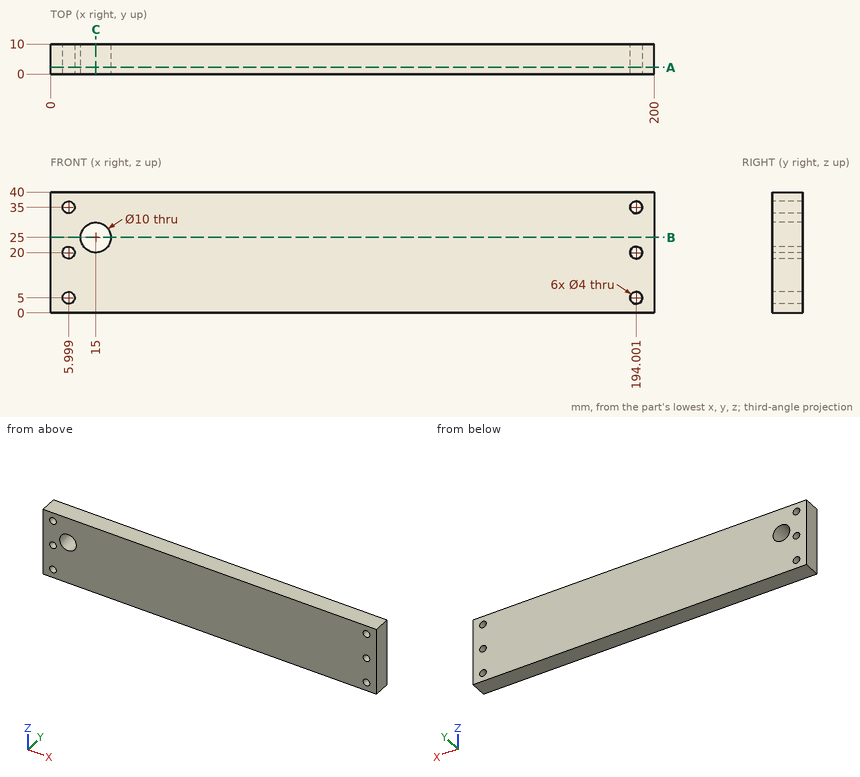
Study the drawing (mm; zero at the part's minimum x, y, z) and answer. Give positions to 0.01 mm unless a question says otherwise; leave off trailing zeros. Write each loop counter-clockwise with the first axis right and the second up, starting at its lowest first coordinate (ties: lowest second). Pieces come first, ordered by that corner, then holes. Notation, with made-up numbers: (-28.75, 36) -> (-6.75, 36) arc R18 ccw to (-6.75, 54) -> close; hole circle Ø6 at (55.25, 29). An arc over 180 degrees is marked (long way). Answer in a Markdown table with one row per item.
1) Section C-C on x = 15 is taken. Give the vertices of the cut face in (y, z).
Results list:
| item | result |
|---|---|
| outline | (0, 0) -> (10, 0) -> (10, 20) -> (0, 20) -> close; (0, 30) -> (10, 30) -> (10, 40) -> (0, 40) -> close |
2) Section B-B on z = 25 is taken. Give the vertices of the cut face in (x, y), plus the area to 3 significant figures.
Results list:
| item | result |
|---|---|
| outline | (0, 0) -> (10, 0) -> (10, 10) -> (0, 10) -> close; (20, 0) -> (200, 0) -> (200, 10) -> (20, 10) -> close |
| area | 1,900 mm^2 |
3) Straight lines are drawn through the part: line 1 (X direction, y = 5.5, z = 3.5) (1 decimal); line 2 (X direction, y = 4.75, z = 35.5) (1 decimal); line 3 (X direction, y = 1.25, z = 29.5). For each, find the intervals that lie inside material, in ascending order. Write a range as [from, to].
Results list:
| item | result |
|---|---|
| line 1 | [0, 4.7], [7.3, 192.7], [195.3, 200] |
| line 2 | [0, 4.1], [7.9, 192.1], [195.9, 200] |
| line 3 | [0, 12.82], [17.18, 200] |
4) Section A-A on y = 2.25 is taken. Give the vertices of the cut face in (x, z).
Results list:
| item | result |
|---|---|
| outline | (0, 0) -> (200, 0) -> (200, 40) -> (0, 40) -> close; hole circle Ø4 at (6, 5); hole circle Ø4 at (6, 20); hole circle Ø4 at (6, 35); hole circle Ø10 at (15, 25); hole circle Ø4 at (194, 5); hole circle Ø4 at (194, 20); hole circle Ø4 at (194, 35) |
5) Each of these flat-tipped pins is pushed along its axis until it touches: pin 1 Ø6 at (y, z) = (5.5, 19) entering from -X; pin 2 Ø3.5 at (x, z) = (6, 35) entering from -Y. Where does it stop, or does it pass through?
Results list:
| item | result |
|---|---|
| pin 1 | x = 0 |
| pin 2 | through |
